Could you check a few things on this model? Use its own coordinates, in mm. A direction names the side the tool comes from. Round coordinates to 2 decimals unless told otherwise and drop trailing zeros. Loops run counter-clockwise (first coordinate to the right, second up) from the corner with the lowest first, then second, coordinate; pieces in that order, holes last. Notation, with made-up numbers: M 61,-24.75 L 71,-24.75 A21 cw 71,-20.75 Z; hole C -6.5,29.5 d4. An arc over 180 degrees is marked long. Answer in a Markdown table with one row per item.
```python
from build123d import *

# Parameters (mm, degrees)
CROQUIS1_R              = 3.5
SALIENTE_EXTRUIR1_DEPTH = 1.5


with BuildPart() as part:
    # Croquis1 → Saliente-Extruir1 (new body)
    with BuildSketch(Plane(origin=(0, 0, 0), x_dir=(-1, 0, 0), z_dir=(0, 0, -1))):
        with BuildLine():
            Line((15.847296355, 27.779408386), (0.694592711, 30.451238869))
            ThreePointArc((0.694592711, 30.451238869), (0, 30.512007857), (-0.694592711, 30.451238869))
            Line((-0.694592711, 30.451238869), (-15.847296355, 27.779408386))
            ThreePointArc((-15.847296355, 27.779408386), (-17.032088886, 27.0953681), (-17.5, 25.80979288))
            Line((-17.5, 25.80979288), (-17.5, -25.487992143))
            ThreePointArc((-17.5, -25.487992143), (-16.914213562, -26.902205705), (-15.5, -27.487992143))
            Line((-15.5, -27.487992143), (15.5, -27.487992143))
            ThreePointArc((15.5, -27.487992143), (16.914213562, -26.902205705), (17.5, -25.487992143))
            Line((17.5, -25.487992143), (17.5, 25.80979288))
            ThreePointArc((17.5, 25.80979288), (17.032088886, 27.0953681), (15.847296355, 27.779408386))
        make_face()
        with Locations(Location((11.25, 7.512007857, 0), (0, 0, 180))):
            Circle(CROQUIS1_R, mode=Mode.SUBTRACT)
        with Locations(Location((11.25, -20.487992143, 0), (0, 0, 180))):
            Circle(CROQUIS1_R, mode=Mode.SUBTRACT)
        with Locations(Location((-11.25, -20.487992143, 0), (0, 0, 180))):
            Circle(CROQUIS1_R, mode=Mode.SUBTRACT)
        with Locations(Location((-11.25, 7.512007857, 0), (0, 0, 180))):
            Circle(CROQUIS1_R, mode=Mode.SUBTRACT)
        with BuildLine():
            Line((-4.75, 14.512007857), (-4.75, 24.512007857))
            ThreePointArc((-4.75, 24.512007857), (-4.164213562, 25.92622142), (-2.75, 26.512007857))
            Line((-2.75, 26.512007857), (2.75, 26.512007857))
            ThreePointArc((2.75, 26.512007857), (4.164213562, 25.92622142), (4.75, 24.512007857))
            Line((4.75, 24.512007857), (4.75, 14.512007857))
            ThreePointArc((4.75, 14.512007857), (3.875930191, 12.859046513), (2.017718795, 12.650888776))
            ThreePointArc((2.017718795, 12.650888776), (0, 13.033559582), (-2.017718795, 12.650888776))
            ThreePointArc((-2.017718795, 12.650888776), (-3.875930191, 12.859046513), (-4.75, 14.512007857))
        make_face(mode=Mode.SUBTRACT)
        with BuildLine():
            Line((4.75, 5.512007857), (4.75, -18.487992143))
            ThreePointArc((4.75, -18.487992143), (4.164213562, -19.902205705), (2.75, -20.487992143))
            Line((2.75, -20.487992143), (-2.75, -20.487992143))
            ThreePointArc((-2.75, -20.487992143), (-4.164213562, -19.902205705), (-4.75, -18.487992143))
            Line((-4.75, -18.487992143), (-4.75, 5.512007857))
            ThreePointArc((-4.75, 5.512007857), (-4.164213562, 6.92622142), (-2.75, 7.512007857))
            Line((-2.75, 7.512007857), (2.75, 7.512007857))
            ThreePointArc((2.75, 7.512007857), (4.164213562, 6.92622142), (4.75, 5.512007857))
        make_face(mode=Mode.SUBTRACT)
        with BuildLine():
            Line((12, -0.487992143), (12, -12.987992143))
            ThreePointArc((12, -12.987992143), (11, -13.987992143), (10, -12.987992143))
            Line((10, -12.987992143), (10, -0.487992143))
            ThreePointArc((10, -0.487992143), (11, 0.512007857), (12, -0.487992143))
        make_face(mode=Mode.SUBTRACT)
        with BuildLine():
            Line((10, 25.512007857), (10, 13.512007857))
            ThreePointArc((10, 13.512007857), (9, 12.512007857), (8, 13.512007857))
            Line((8, 13.512007857), (8, 25.512007857))
            ThreePointArc((8, 25.512007857), (9, 26.512007857), (10, 25.512007857))
        make_face(mode=Mode.SUBTRACT)
        with BuildLine():
            Line((-10, -0.487992143), (-10, -12.987992143))
            ThreePointArc((-10, -12.987992143), (-11, -13.987992143), (-12, -12.987992143))
            Line((-12, -12.987992143), (-12, -0.487992143))
            ThreePointArc((-12, -0.487992143), (-11, 0.512007857), (-10, -0.487992143))
        make_face(mode=Mode.SUBTRACT)
        with BuildLine():
            Line((-8, 25.512007857), (-8, 13.512007857))
            ThreePointArc((-8, 13.512007857), (-9, 12.512007857), (-10, 13.512007857))
            Line((-10, 13.512007857), (-10, 25.512007857))
            ThreePointArc((-10, 25.512007857), (-9, 26.512007857), (-8, 25.512007857))
        make_face(mode=Mode.SUBTRACT)
    extrude(amount=-SALIENTE_EXTRUIR1_DEPTH)


solid = part.part
```
1) I need wall thicknesses on line 1 (X direction, y = -2.5, z = 0.65); line 2 (X direction, y = 13.5, z = 0.15); line 3 (Y direction, x = -11.25, z = 0.75). Which ranges of each line are inside material? Lowest first, please.
Computed:
| item | result |
|---|---|
| line 1 | x = -17.5 to -12, -10 to -4.75, 4.75 to 10, 12 to 17.5 |
| line 2 | x = -17.5 to -10, -8 to -4.48, 4.48 to 8, 10 to 17.5 |
| line 3 | y = -27.49 to -23.99, -16.99 to -13.96, 0.48 to 4.01, 11.01 to 28.59 |
2) I want a section at B-B, the plane x = 11.25. Please give me the cut outline in (y, z).
Computed:
| item | result |
|---|---|
| outline | M -27.49,0 L -23.99,0 L -23.99,1.5 L -27.49,1.5 Z; M -16.99,0 L -13.96,0 L -13.96,1.5 L -16.99,1.5 Z; M 0.48,0 L 4.01,0 L 4.01,1.5 L 0.48,1.5 Z; M 11.01,0 L 28.59,0 L 28.59,1.5 L 11.01,1.5 Z |
3) I want a section at C-C, the plane z = 0.45. State how many separate pieces and enclosed holes the cut face has, plus the area to 3 significant figures.
Computed:
| item | result |
|---|---|
| separate pieces | 1 |
| enclosed holes | 10 |
| area | 1,320 mm² |
4) Which directions (+Z, -Z, +X, -X, +Y, -Y) give clear straight access to the entire face, cutting with the end or side of a thin tool? Please do faces 3 (the face through (-9.022, 12.512, 0.74)), 4 (the face through (8.165, 29.134, 0.74)).
Computed:
| item | result |
|---|---|
| face 3 | +Z, -Z |
| face 4 | +Z, -Z, +X, +Y |
5) I want a section at A-A, the plane y = 15.5. Please give me the cut outline in (x, z).
Computed:
| item | result |
|---|---|
| outline | M -17.5,0 L -10,0 L -10,1.5 L -17.5,1.5 Z; M -8,0 L -4.75,0 L -4.75,1.5 L -8,1.5 Z; M 4.75,0 L 8,0 L 8,1.5 L 4.75,1.5 Z; M 10,0 L 17.5,0 L 17.5,1.5 L 10,1.5 Z |
6) If we mould it in two halves opening along Y, with no side actions, what happens to faces 1 (the face through (17.02, 27.11, 0.74)), 2 (the face through (4.75, 19, 1))? For each: released by +Y, released by -Y, zero draft, split by the parting line, or undercut.
Computed:
| item | result |
|---|---|
| face 1 | released by +Y |
| face 2 | undercut |
